```python
from build123d import *

# Parameters (mm, degrees)
SKETCH1_R          = 13.25
SKETCH1_R_2        = 4.5
BASE_EXTRUDE_DEPTH = 10


with BuildPart() as part:
    # Sketch1 → Base-Extrude (new body)
    with BuildSketch(Plane.XY):
        with BuildLine():
            Line((45.466783574, -8.373426859), (23.737112795, -22.560140288))
            ThreePointArc((23.737112795, -22.560140288), (19.814664383, -24.377101661), (15.536937435, -25))
            Line((15.536937435, -25), (-15, -25))
            ThreePointArc((-15, -25), (-25.606601718, -20.606601718), (-30, -10))
            Line((-30, -10), (-30, 7.67458006))
            ThreePointArc((-30, 7.67458006), (-29.644440107, 10.921174269), (-28.594616806, 14.013853986))
            Line((-28.594616806, 14.013853986), (13.724668775, 104.767854785))
            ThreePointArc((13.724668775, 104.767854785), (14.831693311, 106.030174337), (16.443592136, 106.5))
            Line((16.443592136, 106.5), (83.088534362, 106.5))
            ThreePointArc((83.088534362, 106.5), (85.653269974, 105.056319774), (85.749566861, 102.11475416))
            Line((85.749566861, 102.11475416), (44.112570075, 22.130827513))
            ThreePointArc((44.112570075, 22.130827513), (42.985058136, 17.295192531), (44.322424369, 12.513341381))
            Line((44.322424369, 12.513341381), (48.660254038, 5))
            ThreePointArc((48.660254038, 5), (49.726532496, -2.322620416), (45.466783574, -8.373426859))
        make_face()
        Circle(SKETCH1_R, mode=Mode.SUBTRACT)
        with Locations((40, 0)):
            Circle(SKETCH1_R_2, mode=Mode.SUBTRACT)
    extrude(amount=BASE_EXTRUDE_DEPTH)


solid = part.part
```
The model under review builds one solid part; all positions refer to its coordinate system, in mm. A direction names the side the tool comes from. Round coordinates to 2 decimals unless told otherwise and drop trailing zeros. Order: outer loops, then holes, each group sorted by start corner. A loop starts at its lowest first (then second) coordinate and runs counter-clockwise, first axis right, second up. Notation, with made-up numbers: M 88,59.25 L 105,59.25 A15 cw 105,67.25 Z; hole C 18,-16 d5. An arc over 180 degrees is marked long. Use a Markdown table: item, result.
1) Wall thickness on line 1 along Y through (x, z) = (40, 6.5); line 2 along Y through (x, z) = (0, 7.5); line 3 along X through (y, z) = (2, 3.25): over which ranges is each line inside the solid? List them lowest first. Write a range as [from, to].
Report:
| item | result |
|---|---|
| line 1 | [-11.94, -4.5], [4.5, 106.5] |
| line 2 | [-25, -13.25], [13.25, 75.34] |
| line 3 | [-30, -13.1], [13.1, 35.97], [44.03, 49.8] |
2) Insertion check: pin 1 (1 mm diameter, centred on y = 65.5, z = 2.5, fed in from +X); pin 2 (4 mm diameter, centred on y = 80.5, z = 3.5, fed in from -X); pin 3 (1 mm diameter, centred on y = 91.5, z = 4.5, fed in from -X). Each pin has a flat end and moves straight along its axis. Give the tip position at first contact, or say it passes through.
Report:
| item | result |
|---|---|
| pin 1 | x = 66.95 |
| pin 2 | x = 1.48 |
| pin 3 | x = 7.3 |
3) Consider section D-D (y = 48.5). Write out the cut boundary in (x, z).
Report:
| item | result |
|---|---|
| outline | M -12.51,0 L 57.84,0 L 57.84,10 L -12.51,10 Z |
4) Draft analysis for pull direction Y (two halves, no side actions). For faces 3 (the face through (42.984, 17.365, 4.93)), 4 (the face through (19.87, -24.36, 4.93)), 5 (the face through (-30, -1, 5)), 6 (the face through (-29.654, 10.876, 4.93)), state which applies: released by +Y, released by -Y, zero draft, split by the parting line, or undercut.
Report:
| item | result |
|---|---|
| face 3 | undercut |
| face 4 | released by -Y |
| face 5 | zero draft |
| face 6 | released by +Y |
5) Consider section C-C (y = -6.5). Write out the cut boundary in (x, z), then the cut area to 3 significant figures.
Report:
| item | result |
|---|---|
| outline | M -30,0 L -11.55,0 L -11.55,10 L -30,10 Z; M 11.55,0 L 47.6,0 L 47.6,10 L 11.55,10 Z |
| area | 545 mm^2 |
6) Consider section A-A (z = 5.25). Write out the cut boundary in (x, y).
Report:
| item | result |
|---|---|
| outline | M -30,-10 A15 ccw -15,-25 L 15.54,-25 A15 ccw 23.74,-22.56 L 45.47,-8.37 A10 ccw 48.66,5 L 44.32,12.51 A10 cw 44.11,22.13 L 85.75,102.11 A3 ccw 83.09,106.5 L 16.44,106.5 A3 ccw 13.72,104.77 L -28.59,14.01 A15 ccw -30,7.67 Z; hole C 0,0 d26.5; hole C 40,0 d9 |
7) Tool access review of faces 1 (the face through (7.123, 11.172, 4.93)), 2 (the face through (46.46, 8.81, 4.93)): name each direction out of +Z, -Z, +X, -X, +Y, -Y from which nothing blocks a thin tool from reaching the whole face with its end or side.
Report:
| item | result |
|---|---|
| face 1 | +Z, -Z |
| face 2 | +Z, -Z, +X |
8) Consider section B-B (x = 0). Write out the cut boundary in (y, z), then the cut area to 3 significant figures.
Report:
| item | result |
|---|---|
| outline | M -25,0 L -13.25,0 L -13.25,10 L -25,10 Z; M 13.25,0 L 75.34,0 L 75.34,10 L 13.25,10 Z |
| area | 738 mm^2 |
